Read the model definition and answer for the solid it produces. Units are mm, in the model's axes. A direction names the side the tool comes from. Give positions to 0.01 mm unless a question says otherwise; leave off trailing zeros. Write each loop counter-clockwise with the first axis right and the second up, starting at its lowest first coordinate (ties: lowest second). Pieces come first, ordered by that corner, then holes. Notation, with made-up numbers: M 21,17.25 L 70,17.25 A12 ccw 70,38.25 Z; hole C 48.25,6 d4. An arc over 180 degrees is marked long. Use a Markdown table: item, result. Add a question column.
Item 1: Given P1, Ø1, axis at y = 1.5, z = -5, coming from the +X side, flat-ended and moving along its own axis, determine where the tip first touches the part or whether it passes through.
Item 2: The mould has two halves that part along Y. Classify faces 3 (the flat face through (2.675, 0, -8)), 4 (the cylindrical face through (0, -4, -8)), 5 (the conical face through (-1.798, -1.648, -1.188)), 6 (the conical face through (-0.132, 0.595, -8.359)): pulls with the +Y half, pulls with the -Y half, needs draft (parallel to the pull), parting line crosses it, or undercut.
Item 3: Consider probe 1 along Z at (x, y) = (-1.2, 2.5); probe 2 along Y at (x, z) = (-1.25, -9.25); probe 3 along Y at (x, z) = (-0.8, -9.5). Determine where each line is inside the solid, lowest interval first. Write a range as [from, to].
Item 4: A cutting plane is placed at B-B on z = -5. Determine the outline of the cut face in (x, y) (3 decimals), then the cut area to 3 significant figures.
Item 5: A cutting plane is placed at A-A on z = -8.5. Determine the outline of the cut face in (x, y) (3 decimals).
Item 6: For faces 1 (the cylindrical face through (-2.04, 1.57, -4.98)), 2 (the flat face through (-2.675, 0, -8)), determine the directions among +Z, -Z, +X, -X, +Y, -Y from which every point of the face is accessible in a straight line to the end or side of a thin tool.
Item 7: A cutting plane is placed at C-C on z = -0.5. Determine the outline of the cut face in (x, y) (1 decimal).
from build123d import *

# Parameters (mm, degrees)
SKETCH2_W          = 2.584728437
SKETCH2_H          = 8.43239663
CUT_EXTRUDE1_DEPTH = 12.489125293


with BuildPart() as part:
    # Sketch1 → Revolve1 (revolve)
    with BuildSketch(Plane(origin=(0, 0, 0), x_dir=(0, 0, -1), z_dir=(1, 0, 0)), mode=Mode.PRIVATE) as revolve1_sk:
        Polygon((0, 0), (0, 2.35), (3, 2.575), (6.9, 2.575), (6.9, 4), (10, 4), (10, 2.25), (7.75, 0), align=None)
    revolve(revolve1_sk.sketch.rotate(Axis((0, 0, 0), (0, 0, -1)), 90), axis=Axis((0, 0, 0), (0, 0, -1)))

    # Sketch2 → Cut-Extrude1 (cut, through all)
    with BuildSketch(Plane(origin=(0, 0, -10), x_dir=(-1, 0, 0), z_dir=(0, 0, -1))):
        with Locations((3.967364219, 0)):
            Rectangle(SKETCH2_W, SKETCH2_H)
        with Locations((-3.967364219, 0)):
            Rectangle(SKETCH2_W, SKETCH2_H)
    extrude(amount=-CUT_EXTRUDE1_DEPTH, mode=Mode.SUBTRACT)


solid = part.part
Filled in:
| question | item | result |
|---|---|---|
| 1 | P1 | x = 2.37 |
| 2 | face 3 | needs draft |
| 2 | face 4 | pulls with the -Y half |
| 2 | face 5 | parting line crosses it |
| 2 | face 6 | undercut |
| 3 | probe 1 | [-10, -6.9] |
| 3 | probe 2 | [-3.8, -0.83], [0.83, 3.8] |
| 3 | probe 3 | [-3.92, -1.56], [1.56, 3.92] |
| 4 | outline | C 0,0 d5.15 |
| 4 | area | 20.8 mm² |
| 5 | outline | M -2.675,-2.974 A4 ccw 2.675,-2.974 L 2.675,2.974 A4 ccw -2.675,2.974 Z; hole C 0,0 d1.5 |
| 6 | face 1 | +Z |
| 6 | face 2 | +Z, -Z, -X, +Y, -Y |
| 7 | outline | C 0,0 d4.8 |
